Here's the drawing with two shaded views (mm, measured from the low corner). I have some questions. A direction names the side the tool comes from. Round coordinates to 2 decimals unless told otherwise and drop trailing zeros. Loops run counter-clockwise (first coordinate to the right, second up) from the corner with the lowest first, then second, coordinate; pieces in that order, holes last. Notation, with made-up numbers: (0.5, 11.5) - (8.5, 11.5) arc R24 ccw to (8.5, 25.5) - close; hole circle Ø10 at (-15.75, -15). An arc over 180 degrees is marked (long way). Answer as CSV lines item,"result".
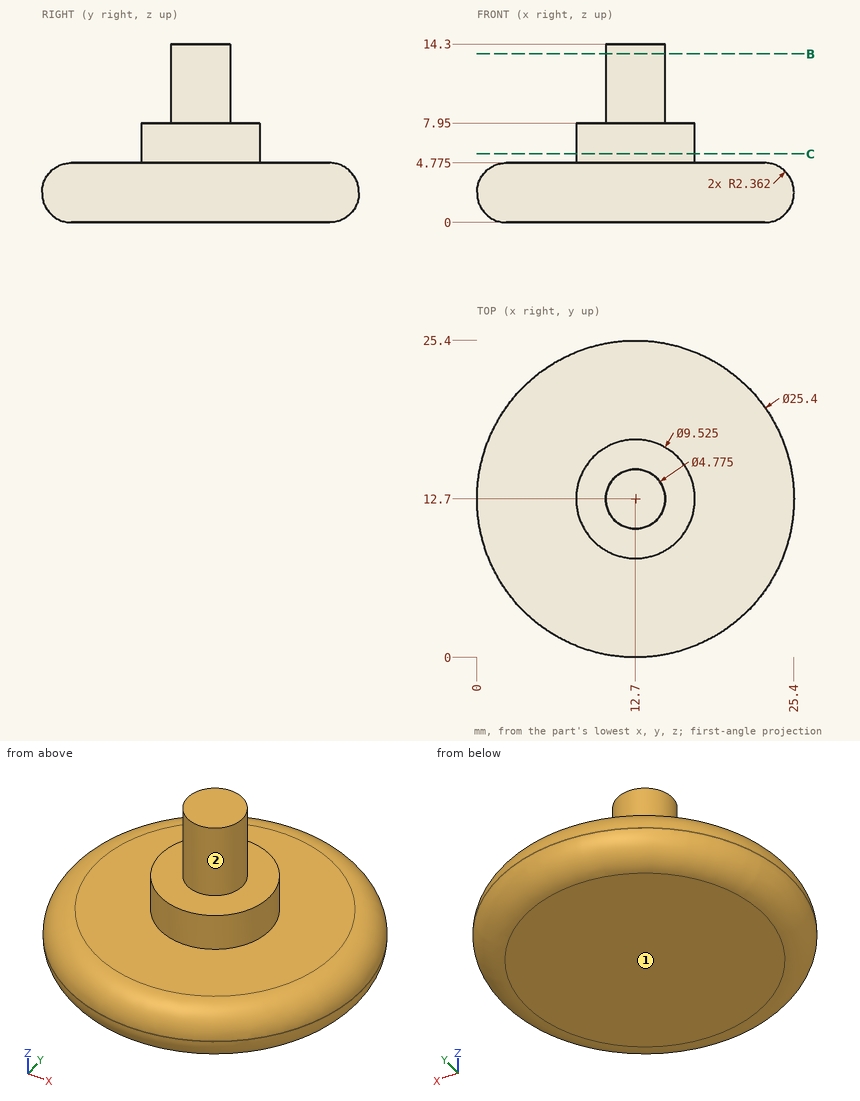
Q1. I'm going to push flat-ended pins straight in: pin 1 Ø1.5 at (x, y) = (3.5, 5) entering from -Z; pin 2 Ø1 at (x, y) = (11.5, 7.5) entering from -Z; pin 3 Ø2 at (x, z) = (21, 2.5) entering from -Y. Where does each tip first touch, or does it pass through?
Checks:
pin 1,"z = 0.18"
pin 2,"z = 0"
pin 3,"y = 2.31"
Q2. If I drill on line 1 along Z through (x, y) = (22.5, 16) (1 decimal); line 2 along Z through (x, y) = (9.5, 9.25); line 3 along Y through (x, z) = (22.25, 2.5), over which ranges is the centre line in solid material (lowest first)? Write a range as [from, to].
Checks:
line 1,"[0, 4.8]"
line 2,"[0, 7.95]"
line 3,"[4.33, 21.07]"
Q3. On a 3-axis mill with a long thin cutter (end or side, diameter ignored), from which of +Z, -Z, +X, -X, +Y, -Y can I reach the whole of each face in a straight line? I mean the marked faces 1 and 2. Say none if no direction works.
Checks:
face 1,"-Z, +X, -X, +Y, -Y"
face 2,"+Z"
Q4. Imagine slicing it at B-B (z = 13.5). Write out the boundary of the cut face in (x, y) (1 decimal).
Checks:
outline,"circle Ø4.8 at (12.7, 12.7)"
Q5. Imagine slicing it at C-C (z = 5.5). Write out the boundary of the cut face in (x, y) (1 decimal).
Checks:
outline,"circle Ø9.5 at (12.7, 12.7)"
